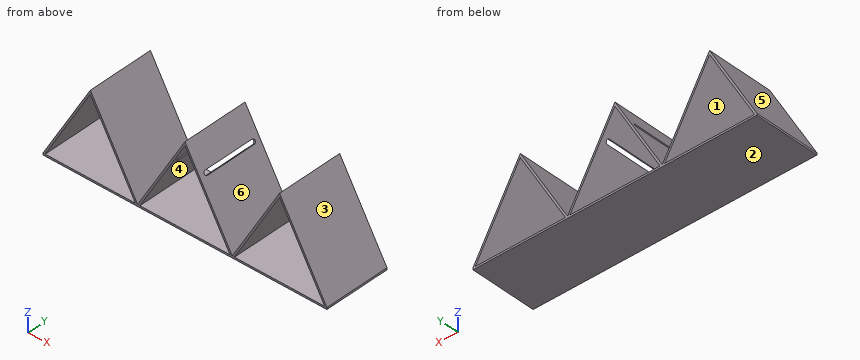
from build123d import *

# Parameters (mm, degrees)
F1_DEPTH = 105
F4_DEPTH = 3
F5_DEPTH = 3.2


with BuildPart() as f1:
    # F0 (on Front) → F1 (new body)
    with BuildSketch(Plane.XZ):
        Polygon((31.5868725905, 38.7087155582), (-43.4131274095, -91.1950950095), (-39.9490257943, -91.1950950095), (31.5868725905, 32.7087155582), (103.1227709754, -91.1950950095), (106.5868725905, -91.1950950095), align=None)
        Polygon((181.5868725905, 38.7087155582), (106.5868725905, -91.1950950095), (110.0509742057, -91.1950950095), (181.5868725905, 32.7087155582), (253.1227709754, -91.1950950095), (256.5868725905, -91.1950950095), align=None)
        Polygon((403.1227709754, -91.1950950095), (406.5868725905, -91.1950950095), (331.5868725905, 38.7087155582), (256.5868725905, -91.1950950095), (260.0509742057, -91.1950950095), (331.5868725905, 32.7087155582), align=None)
        Polygon((-39.9490257943, -91.1950950095), (-43.4131274095, -91.1950950095), (-43.3987992861, -94.1795955126), (406.5868725905, -94.1795955126), (406.5868725905, -91.1950950095), (403.1227709754, -91.1950950095), (260.0509742057, -91.1950950095), (256.5868725905, -91.1950950095), (253.1227709754, -91.1950950095), (110.0509742057, -91.1950950095), (106.5868725905, -91.1950950095), (103.1227709754, -91.1950950095), align=None)
    extrude(amount=F1_DEPTH)

    # F2 (on face) → F4 (cut)
    with BuildSketch(Plane(origin=(152.9515199535, 0, 88.3066012181), x_dir=(0, 1, 0), z_dir=(0.8660254038, 0, 0.5))):
        with BuildLine():
            Line((-11.2848039716, -100.270705274), (-93.8924178481, -100.270705274))
            ThreePointArc((-93.8924178481, -100.270705274), (-97, -103.770705274), (-93.8924178481, -107.270705274))
            Line((-93.8924178481, -107.270705274), (-10.656950064, -107.270705274))
            ThreePointArc((-10.656950064, -107.270705274), (-8.0142508316, -103.5055153734), (-11.2848039716, -100.270705274))
        make_face()
    extrude(amount=-F4_DEPTH, mode=Mode.SUBTRACT)

    # F3 (on face) → F5 (cut)
    with BuildSketch(Plane(origin=(119.4287889323, 0, -68.952243439), x_dir=(0, -1, 0), z_dir=(-0.8660254038, 0, 0.5))):
        with BuildLine():
            Line((93.957901001, 81.3161673165), (10.8784036711, 81.3161673165))
            ThreePointArc((10.8784036711, 81.3161673165), (8.0006789358, 77.7585614935), (11.0152736306, 74.3161673165))
            Line((11.0152736306, 74.3161673165), (94.2316353321, 74.3161673165))
            ThreePointArc((94.2316353321, 74.3161673165), (96.9972779307, 77.9296696835), (93.957901001, 81.3161673165))
        make_face()
    extrude(amount=-F5_DEPTH, mode=Mode.SUBTRACT)


solid = f1.part
Build history of the part. All positions in model axes, mm. Face numbers are marked on the shaded views. A direction names the side the tool comes from. Give positions to 0.01 mm unless a question says otherwise; leave off trailing zeros. Write each loop counter-clockwise with the first axis right and the second up, starting at its lowest first coordinate (ties: lowest second). Pieces come first, ordered by that corner, then holes. Notation, with made-up numbers: (50.25, 22) - (54.25, 22) arc R9 ccw to (54.25, 33) - close; hole circle Ø5 at (-39, 7). An arc over 180 degrees is marked (long way). Use one line per item in the form item = value. Start each with the question number.
1. Two-plate mould, pull along Z, no slides. Class the marked faces 1, 2 and 3: released by +Z, released by -Z, zero draft, split by the parting line, or undercut.
2. Band-saw the part on B-B on z = -72. Write the cut outline in (x, y), plus the area to 3 significant figures.
3. Drop flat-ended pins along their axis: pin 1 Ø6 at (x, y) = (57, -42) entering from +Z; pin 2 Ø3 at (x, y) = (261, -13.5) entering from +Z; pin 3 Ø6 at (x, y) = (14, -40) entering from +Z. Give the stop position or say it passes through.
4. Probe line 1 (X direction, y = -83.5, z = -29); line 2 (X direction, y = -92, z = -61); line 3 (Z direction, x = 120, y = -55.5). List the from-to ranges inside material, lowest first. Write a range as [from, to].
5. Band-saw the part on A-A on y = -65. Write the cut outline in (x, z).
6. 3-axis set-ups, long thin cutter, end or side, ignore diameter. For the marked faces 4, 5 and 6: which of +Z, -Z, +X, -X, +Y, -Y reach the whole face in a straight line?
7. Band-saw the part on C-C on x = 343. Write the cut outline in (y, z).
Conclusion:
q1.face_1 = undercut
q1.face_2 = released by -Z
q1.face_3 = released by +Z
q2.outline = (-32.33, -105) - (-28.87, -105) - (-28.87, 0) - (-32.33, 0) - close; (92.04, -105) - (95.5, -105) - (95.5, 0) - (92.04, 0) - close; (117.67, -105) - (121.13, -105) - (121.13, 0) - (117.67, 0) - close; (242.04, -105) - (245.5, -105) - (245.5, 0) - (242.04, 0) - close; (267.67, -105) - (271.13, -105) - (271.13, 0) - (267.67, 0) - close; (392.04, -105) - (395.5, -105) - (395.5, 0) - (392.04, 0) - close
q2.area = 2,180 mm²
q3.pin_1 = -0.11
q3.pin_2 = -80.95
q3.pin_3 = 13.44
q4.line_1 = [-7.5, -4.04], [67.21, 70.68], [142.5, 145.96], [217.21, 220.68], [292.5, 295.96], [367.21, 370.68]
q4.line_2 = [-25.98, -22.52], [85.69, 89.15], [124.02, 127.48], [235.69, 239.15], [274.02, 277.48], [385.69, 389.15]
q4.line_3 = [-94.18, -91.2], [-73.96, -67.96]
q5.outline = (-43.41, -91.2) - (-43.4, -94.18) - (406.59, -94.18) - (406.59, -91.2) - (331.59, 38.71) - (256.59, -91.2) - (206.59, -4.59) - (203.99, -6.09) - (253.12, -91.2) - (110.05, -91.2) - (159.18, -6.09) - (156.59, -4.59) - (106.59, -91.2) - (31.59, 38.71) - close; (160.09, 1.47) - (162.68, -0.03) - (181.59, 32.71) - (200.49, -0.03) - (203.09, 1.47) - (181.59, 38.71) - close; hole (-39.95, -91.2) - (103.12, -91.2) - (31.59, 32.71) - close; hole (260.05, -91.2) - (403.12, -91.2) - (331.59, 32.71) - close
q6.face_4 = +Y, -Y
q6.face_5 = +Z, -X, +Y, -Y
q6.face_6 = +Z, +Y, -Y
q7.outline = (-105, -94.18) - (0, -94.18) - (0, -91.2) - (-105, -91.2) - close; (-105, 12.94) - (0, 12.94) - (0, 18.94) - (-105, 18.94) - close
